```python
from build123d import *

# Parameters (mm, degrees)
F0_W         = 150
F0_H         = 118
F0_W_2       = 5
F0_H_2       = 5
F0_R         = 7.5
F0_R_2       = 12
F1_DEPTH     = 5
F2_DEPTH     = 1
F3_SIZE      = 0.5
F4_T1_DEPTH  = 160
F4_T3_DEPTH  = 128
F5_T1_DEPTH  = 8
F5_S5_W      = 2
F5_S5_H      = 2
F5_T6_DEPTH  = 2
F5_S11_W     = 2
F5_S11_H     = 2
F5_T12_DEPTH = 2
F5_S17_W     = 2
F5_S17_H     = 2
F5_T18_DEPTH = 2
F5_S23_W     = 2
F5_S23_H     = 2
F5_T24_DEPTH = 2


# Not quite as in the source:
# - a fillet or chamfer that OpenCascade refuses, or shapes differently, is made with other operations: its cross-section is extruded or revolved along the edge and cut away or added


with BuildPart() as f1:
    # F0 (on Top) → F1 (new body)
    with BuildSketch(Plane.XY):
        with Locations((0.2827864019, -6.098040469)):
            Rectangle(F0_W, F0_H)
        with Locations((-67.2172135981, -57.598040469)):
            Rectangle(F0_W_2, F0_H_2, mode=Mode.SUBTRACT)
        with Locations((-55.7172135981, -46.098040469)):
            Circle(F0_R, mode=Mode.SUBTRACT)
        with Locations((-27.7172135981, -46.098040469)):
            Circle(F0_R, mode=Mode.SUBTRACT)
        with Locations((0.2827864019, -46.098040469)):
            Circle(F0_R, mode=Mode.SUBTRACT)
        with Locations((28.2827864019, -46.098040469)):
            Circle(F0_R, mode=Mode.SUBTRACT)
        with Locations((67.7827864019, -57.598040469)):
            Rectangle(F0_W_2, F0_H_2, mode=Mode.SUBTRACT)
        with Locations((56.2827864019, -46.098040469)):
            Circle(F0_R, mode=Mode.SUBTRACT)
        with Locations((-67.2172135981, 45.401959531)):
            Rectangle(F0_W_2, F0_H_2, mode=Mode.SUBTRACT)
        with Locations((0.2827864019, 12.901959531)):
            Circle(F0_R_2, mode=Mode.SUBTRACT)
        with Locations((67.7827864019, 45.401959531)):
            Rectangle(F0_W_2, F0_H_2, mode=Mode.SUBTRACT)
        with Locations((-67.2172135981, -57.598040469)):
            Rectangle(F0_W_2, F0_H_2)
        with Locations((-67.2172135981, 45.401959531)):
            Rectangle(F0_W_2, F0_H_2)
        with Locations((67.7827864019, 45.401959531)):
            Rectangle(F0_W_2, F0_H_2)
        with Locations((67.7827864019, -57.598040469)):
            Rectangle(F0_W_2, F0_H_2)
    extrude(amount=F1_DEPTH)

    # F0 (on Top) → F2 (cut)
    with BuildSketch(Plane.XY):
        with Locations((-67.2172135981, 45.401959531)):
            Rectangle(F0_W_2, F0_H_2)
        with Locations((67.7827864019, 45.401959531)):
            Rectangle(F0_W_2, F0_H_2)
        with Locations((67.7827864019, -57.598040469)):
            Rectangle(F0_W_2, F0_H_2)
        with Locations((-67.2172135981, -57.598040469)):
            Rectangle(F0_W_2, F0_H_2)
    extrude(amount=F2_DEPTH, mode=Mode.SUBTRACT)

    # F3
    f3_edges = [f1.edges().sort_by_distance(p)[0] for p in [
        (-11.717214, 12.90196, 5),
        (-63.217214, -46.09804, 5),
        (-35.217214, -46.09804, 5),
        (-7.217214, -46.09804, 5),
        (20.782786, -46.09804, 5),
        (48.782786, -46.09804, 5),
    ]]
    chamfer(f3_edges, length=F3_SIZE)

    # F4: fillet of radius 2 on 10 edges, made by hand

    # F4_s2 → F4_t1 (cut)
    with BuildSketch(Plane.YZ.offset(-79.7172135981)):
        with BuildLine():
            ThreePointArc((50.901959531, 5), (52.3161730933, 4.4142135624), (52.901959531, 3))
            Line((52.901959531, 3), (52.901959531, 5))
            Line((52.901959531, 5), (50.901959531, 5))
        make_face()
        with BuildLine():
            ThreePointArc((-63.098040469, 5), (-64.5122540314, 4.4142135624), (-65.098040469, 3))
            Line((-65.098040469, 3), (-65.098040469, 5))
            Line((-65.098040469, 5), (-63.098040469, 5))
        make_face()
    extrude(amount=F4_T1_DEPTH, mode=Mode.SUBTRACT)

    # F4_s4 → F4_t3 (cut)
    with BuildSketch(Plane.XZ.offset(-57.901959531)):
        with BuildLine():
            ThreePointArc((-72.7172135981, 5), (-74.1314271605, 4.4142135624), (-74.7172135981, 3))
            Line((-74.7172135981, 3), (-74.7172135981, 5))
            Line((-74.7172135981, 5), (-72.7172135981, 5))
        make_face()
        with BuildLine():
            ThreePointArc((73.2827864019, 5), (74.6969999642, 4.4142135624), (75.2827864019, 3))
            Line((75.2827864019, 3), (75.2827864019, 5))
            Line((75.2827864019, 5), (73.2827864019, 5))
        make_face()
    extrude(amount=F4_T3_DEPTH, mode=Mode.SUBTRACT)

    # F4_s5 → F4_t6 (revolve, cut)
    with BuildSketch(Plane.XZ.offset(-12.901959531)):
        with BuildLine():
            ThreePointArc((13.6056620574, 5), (12.8985552762, 4.8708286934), (12.2827864019, 4.5))
            Line((12.2827864019, 4.5), (12.7827864019, 5))
            Line((12.7827864019, 5), (13.6056620574, 5))
        make_face()
    revolve(axis=Axis((0.2827864019, 12.901959531, 5), (0, 0, 1)), mode=Mode.SUBTRACT)

    # F4_s7 → F4_t8 (revolve, cut)
    with BuildSketch(Plane.XZ.offset(46.098040469)):
        with BuildLine():
            ThreePointArc((-46.8943379426, 5), (-47.6014447238, 4.8708286934), (-48.2172135981, 4.5))
            Line((-48.2172135981, 4.5), (-47.7172135981, 5))
            Line((-47.7172135981, 5), (-46.8943379426, 5))
        make_face()
    revolve(axis=Axis((-55.7172135981, -46.098040469, 5), (0, 0, 1)), mode=Mode.SUBTRACT)

    # F4_s9 → F4_t10 (revolve, cut)
    with BuildSketch(Plane.XZ.offset(46.098040469)):
        with BuildLine():
            ThreePointArc((-18.8943379426, 5), (-19.6014447238, 4.8708286934), (-20.2172135981, 4.5))
            Line((-20.2172135981, 4.5), (-19.7172135981, 5))
            Line((-19.7172135981, 5), (-18.8943379426, 5))
        make_face()
    revolve(axis=Axis((-27.7172135981, -46.098040469, 5), (0, 0, 1)), mode=Mode.SUBTRACT)

    # F4_s11 → F4_t12 (revolve, cut)
    with BuildSketch(Plane.XZ.offset(46.098040469)):
        with BuildLine():
            ThreePointArc((9.1056620574, 5), (8.3985552762, 4.8708286934), (7.7827864019, 4.5))
            Line((7.7827864019, 4.5), (8.2827864019, 5))
            Line((8.2827864019, 5), (9.1056620574, 5))
        make_face()
    revolve(axis=Axis((0.2827864019, -46.098040469, 5), (0, 0, 1)), mode=Mode.SUBTRACT)

    # F4_s13 → F4_t14 (revolve, cut)
    with BuildSketch(Plane.XZ.offset(46.098040469)):
        with BuildLine():
            ThreePointArc((37.1056620574, 5), (36.3985552762, 4.8708286934), (35.7827864019, 4.5))
            Line((35.7827864019, 4.5), (36.2827864019, 5))
            Line((36.2827864019, 5), (37.1056620574, 5))
        make_face()
    revolve(axis=Axis((28.2827864019, -46.098040469, 5), (0, 0, 1)), mode=Mode.SUBTRACT)

    # F4_s15 → F4_t16 (revolve, cut)
    with BuildSketch(Plane.XZ.offset(46.098040469)):
        with BuildLine():
            ThreePointArc((65.1056620574, 5), (64.3985552762, 4.8708286934), (63.7827864019, 4.5))
            Line((63.7827864019, 4.5), (64.2827864019, 5))
            Line((64.2827864019, 5), (65.1056620574, 5))
        make_face()
    revolve(axis=Axis((56.2827864019, -46.098040469, 5), (0, 0, 1)), mode=Mode.SUBTRACT)

    # F5: fillet of radius 2 on 14 edges, made by hand

    # F5_s2 → F5_t1 (cut)
    with BuildSketch(Plane.XY.offset(-5)):
        with BuildLine():
            ThreePointArc((73.2827864019, -65.098040469), (74.6969999642, -64.5122540314), (75.2827864019, -63.098040469))
            Line((75.2827864019, -63.098040469), (75.2827864019, -65.098040469))
            Line((75.2827864019, -65.098040469), (73.2827864019, -65.098040469))
        make_face()
        with BuildLine():
            ThreePointArc((-72.7172135981, -65.098040469), (-74.1314271605, -64.5122540314), (-74.7172135981, -63.098040469))
            Line((-74.7172135981, -63.098040469), (-74.7172135981, -65.098040469))
            Line((-74.7172135981, -65.098040469), (-72.7172135981, -65.098040469))
        make_face()
        with BuildLine():
            ThreePointArc((-74.7172135981, 50.901959531), (-74.1314271605, 52.3161730933), (-72.7172135981, 52.901959531))
            Line((-72.7172135981, 52.901959531), (-74.7172135981, 52.901959531))
            Line((-74.7172135981, 52.901959531), (-74.7172135981, 50.901959531))
        make_face()
        with BuildLine():
            ThreePointArc((75.2827864019, 50.901959531), (74.6969999642, 52.3161730933), (73.2827864019, 52.901959531))
            Line((73.2827864019, 52.901959531), (75.2827864019, 52.901959531))
            Line((75.2827864019, 52.901959531), (75.2827864019, 50.901959531))
        make_face()
    extrude(amount=F5_T1_DEPTH, mode=Mode.SUBTRACT)


with BuildPart() as f5_tool4:
    # F5_s5 → F5_t6 (new body)
    with BuildSketch(Plane.YZ.offset(73.2827864019)):
        with Locations((51.901959531, 4)):
            Rectangle(F5_S5_W, F5_S5_H)
    extrude(amount=F5_T6_DEPTH)

    # F5_s7 → F5_t8 (revolve, cut)
    with BuildSketch(Plane(origin=(73.2827864019, 50.901959531, 3), x_dir=(0, -0.7071067812, -0.7071067812), z_dir=(0, -0.7071067812, 0.7071067812))):
        with BuildLine():
            ThreePointArc((0, -2), (2, 0), (0, 2))
            Line((0, 2), (0, -2))
        make_face()
    revolve(axis=Axis((73.2827864019, 50.901959531, 3), (1, 0, 0)), mode=Mode.SUBTRACT)


with BuildPart() as f1_1:
    add(f1.part)

    # F5_t3: cut F5_tool4
    add(f5_tool4.part, mode=Mode.SUBTRACT)


with BuildPart() as f5_tool10:
    # F5_s11 → F5_t12 (new body)
    with BuildSketch(Plane.XZ.offset(63.098040469)):
        with Locations((74.2827864019, 4)):
            Rectangle(F5_S11_W, F5_S11_H)
    extrude(amount=F5_T12_DEPTH)

    # F5_s13 → F5_t14 (revolve, cut)
    with BuildSketch(Plane(origin=(73.2827864019, -63.098040469, 3), x_dir=(-0.7071067812, 0, -0.7071067812), z_dir=(-0.7071067812, 0, 0.7071067812))):
        with BuildLine():
            ThreePointArc((0, -2), (2, 0), (0, 2))
            Line((0, 2), (0, -2))
        make_face()
    revolve(axis=Axis((73.2827864019, -63.098040469, 3), (0, -1, 0)), mode=Mode.SUBTRACT)


with BuildPart() as f1_2:
    add(f1_1.part)

    # F5_t9: cut F5_tool10
    add(f5_tool10.part, mode=Mode.SUBTRACT)


with BuildPart() as f5_tool16:
    # F5_s17 → F5_t18 (new body)
    with BuildSketch(Plane.XZ.offset(63.098040469)):
        with Locations((-73.7172135981, 4)):
            Rectangle(F5_S17_W, F5_S17_H)
    extrude(amount=F5_T18_DEPTH)

    # F5_s19 → F5_t20 (revolve, cut)
    with BuildSketch(Plane(origin=(-72.7172135981, -63.098040469, 3), x_dir=(0.7071067812, 0, -0.7071067812), z_dir=(-0.7071067812, 0, -0.7071067812))):
        with BuildLine():
            ThreePointArc((0, -2), (2, 0), (0, 2))
            Line((0, 2), (0, -2))
        make_face()
    revolve(axis=Axis((-72.7172135981, -63.098040469, 3), (0, -1, 0)), mode=Mode.SUBTRACT)


with BuildPart() as f1_3:
    add(f1_2.part)

    # F5_t15: cut F5_tool16
    add(f5_tool16.part, mode=Mode.SUBTRACT)


with BuildPart() as f5_tool22:
    # F5_s23 → F5_t24 (new body)
    with BuildSketch(Plane.YZ.offset(-72.7172135981)):
        with Locations((51.901959531, 4)):
            Rectangle(F5_S23_W, F5_S23_H)
    extrude(amount=-F5_T24_DEPTH)

    # F5_s25 → F5_t26 (revolve, cut)
    with BuildSketch(Plane(origin=(-72.7172135981, 50.901959531, 3), x_dir=(0, -0.7071067812, -0.7071067812), z_dir=(0, 0.7071067812, -0.7071067812))):
        with BuildLine():
            ThreePointArc((0, -2), (2, 0), (0, 2))
            Line((0, 2), (0, -2))
        make_face()
    revolve(axis=Axis((-72.7172135981, 50.901959531, 3), (-1, 0, 0)), mode=Mode.SUBTRACT)


with BuildPart() as f1_4:
    add(f1_3.part)

    # F5_t21: cut F5_tool22
    add(f5_tool22.part, mode=Mode.SUBTRACT)


solid = f1_4.part
```
Input: part model. Units: mm. Frame: model coordinates. A direction names the side the tool comes from. Coordinates: 2 decimals unless noted, no trailing zeros. Answer in a Markdown table with one row per item.
1. First-contact query: pin 1 (17 mm diameter, centred on x = 56.28, y = -46.1, fed in from +Z); pin 2 (9 mm diameter, centred on x = 28.28, y = -46.1, fed in from +Z); pin 3 (4 mm diameter, centred on x = -67.5, y = 45, fed in from -Z). Flat tips, straight axial feed; report the tip coordinate or a pass-through.
Response:
| item | result |
|---|---|
| pin 1 | stops at z = 4.97 |
| pin 2 | passes through |
| pin 3 | stops at z = 1 |
2. Reachability of faces 1 (the cylindrical face through (4.31, -39.77, 2.22)), 2 (the flat face through (68, 45, 1)) from +Z, -Z, +X, -X, +Y, -Y: full face, straight path, thin tool, end or side. Return the list, or none.
Response:
| item | result |
|---|---|
| face 1 | +Z, -Z |
| face 2 | -Z |
3. Material intervals for line 1 (Y direction, x = 0, z = 1.9); line 2 (X direction, y = -46, z = 1.8); line 3 (Y direction, x = 5, z = 2.8), sorted ascending.
Response:
| item | result |
|---|---|
| line 1 | y = -65.1 to -53.59, -38.6 to 0.91, 24.9 to 52.9 |
| line 2 | x = -74.72 to -63.22, -48.22 to -35.22, -20.22 to -7.22, 7.78 to 20.78, 35.78 to 48.78, 63.78 to 75.28 |
| line 3 | y = -65.1 to -51.93, -40.27 to 1.87, 23.94 to 52.9 |
4. Section A-A, the plane x = -4.5. Count the separate pieces of the cut face and the enclosed holes in it, then the cut area to 3 significant figures.
Response:
| item | result |
|---|---|
| separate pieces | 3 |
| enclosed holes | 0 |
| area | 419 mm2 |
5. Draft query along X for faces 3 (the flat face through (-67, 45, 1)), 4 (the flat face through (-74.717, -7, 1)), 5 (the flat face through (-1, 52.902, 1)). Return one class per face: pulls with the +X half, pulls with the -X half, needs draft (parallel to the pull), parting line crosses it, or undercut.
Response:
| item | result |
|---|---|
| face 3 | undercut |
| face 4 | pulls with the -X half |
| face 5 | needs draft |
